Autodesk Inventor part; units mm, degrees
ref_plane "YZ Plane" through (0, 0, 0) normal (1, 0, 0) x (0, 1, 0)
ref_plane "XZ Plane" through (0, 0, 0) normal (0, 1, 0) x (-1, 0, 0)
ref_plane "XY Plane" through (0, 0, 0) normal (0, 0, 1) x (1, 0, 0)
sketch "Szkic1" plane through (0, 0, 0) normal (0, 1, 0) x (-1, 0, 0)
  line L0 (-125.2393, -14.1807) -> (-26.2247, 164.0455)
  arc A0 (-125.2393, -14.1807) -> (-99.0146, -58.75) centre (-99.0146, -28.75) ccw
  line L1 (99.0146, -58.75) -> (-99.0146, -58.75)
  line L2 (26.2247, 164.0455) -> (125.2393, -14.1807)
  arc A1 (26.2247, 164.0455) -> (-26.2247, 164.0455) centre (0, 149.4762) ccw
  line L3 (-23.6022, 162.5886) -> (-122.6168, -15.6376)
  arc A2 (-122.6168, -15.6376) -> (-99.0146, -55.75) centre (-99.0146, -28.75) ccw
  line L4 (-99.0146, -55.75) -> (99.0146, -55.75)
  arc A3 (113.6938, -51.4109) -> (125.9544, -30.5508) centre (99.0146, -28.75) ccw
  line L5 (122.6168, -15.6376) -> (23.6022, 162.5886)
  arc A4 (23.6022, 162.5886) -> (-23.6022, 162.5886) centre (0, 149.4762) ccw
  circle A5 centre (99.0146, -28.75) radius 5.1
  arc A6 (104.1146, -20.1483) -> (94.9151, -37.8711) centre (99.0146, -28.75) ccw
  line L6 (104.1146, -20.1483) -> (125.9544, -30.5508)
  line L7 (94.9151, -37.8711) -> (113.6938, -51.4109)
  arc A7 (99.0146, -58.75) -> (116.2857, -53.2797) centre (99.0146, -28.75) ccw
  arc A8 (128.8458, -31.9279) -> (125.2393, -14.1807) centre (99.0146, -28.75) ccw
  point P0 (0, 0)
  point P1 (0, 0)
  dimension "d0" = 3
  dimension "d1" = 10.2
  dimension "d2" = 20
extrude "Wyciągnięcie proste1" add sketch "Szkic1" along normal blind 5
sketch "Szkic2" plane through (0, 5, 0) normal (0, 1, 0) x (1, 0, 0)
  circle A0 centre (-99.0146, 28.75) radius 5.1
  circle A1 centre (-99.0146, 28.75) radius 5.1
  point P0 (0, 0)
extrude "Wyciągnięcie proste2" add sketch "Szkic2" against normal blind 5
sketch "Szkic3" plane through (0, 5, 0) normal (0, 1, 0) x (1, 0, 0)
  arc A0 (-104.1146, 20.1483) -> (-94.9151, 37.8711) centre (-99.0146, 28.75) ccw
  circle A1 centre (-99.0146, 28.75) radius 5.1
  circle A2 centre (-99.0146, 28.75) radius 10
  point P0 (0, 0)
  point P1 (-94.9151, 37.8711)
  dimension "d7" = 10.2
extrude "Wyciągnięcie proste3" add sketch "Szkic3" along normal blind 1
fillet "Zaokrąglenie1" radius 2 1 edges at (-107.8901, 5, -33.357)
sketch "Szkic4" plane through (0, 0, 0) normal (0, -1, 0) x (1, 0, 0)
  line L0 (-94.9151, -37.8711) -> (-113.6938, -51.4109)
  arc A0 (-94.9151, -37.8711) -> (-104.1146, -20.1483) centre (-99.0146, -28.75) ccw
  line L1 (-125.9544, -30.5508) -> (-104.1146, -20.1483)
  arc A1 (-125.9544, -30.5508) -> (-113.6938, -51.4109) centre (-99.0146, -28.75) ccw
  point P0 (0, 0)
extrude "Wyciągnięcie proste4" add sketch "Szkic4" along normal blind 15
properties part number "_Drukowanie 3D"
The listing builds one solid part. Answer for the finished solid, in the listing's coordinates (mm). A direction names the side the tool comes from. Coordinates: 2 decimals unless noted, no trailing zeros. Loops run counter-clockwise (first coordinate to the right, second up) from the corner with the lowest first, then second, coordinate; pieces in that order, holes last.
1) Find section C-C on y = -7. Write down the section's boundary in (x, z).
2) Find section A-A on z = -28.75. Write down the section's boundary in (x, y).
3) Find section B-B on x = -117.5. Write down the section's boundary in (y, z).
4) A tool of negligible diameter and unlimited length cuts with its end or side. For faces 4 (the face through (-104.173, -4.647, -44.546)), 5 (the face through (-99, 5, -29)), from which of +Z, -Z, +X, -X, +Y, -Y can it reach the whole face along a straight path? Write none if from no direction.
5) Determine the mould class of faces 1 (the face through (-115, 5, -37)), 2 (the face through (-114.882, -4.647, -25.277)), 3 (the face through (-108, -15, -35)) for opening direction Y: pulls with the +Y half, pulls with the -Y half, needs draft (parallel to the pull), parting line crosses it, or undercut.
6) Find the intervals of material crossed by L1, parallel to Y at x = -113.5, z = -29.5; L2, parallel to X at y = 5.7, z = -28.75; L3, parallel to X at y = 5.5, z = -28.75, in increasing order.
7) Find section D-D on z = -41. Write down the section's boundary in (x, y), then the cut area to 3 significant figures.
8) Flat-ended cylindrical pins translate along their axes: pin 1 Ø2 at (y, z) = (-8.5, -43.5) entering from +X; pin 2 Ø3 at (x, y) = (-93, 2.5) entering from +Z; pin 3 Ø3 at (x, z) = (-98.5, -29) entering from +Y. Find the tip coordinate at first contact, or state that the pin passes through.
Values:
1. outline: (-125.95, -30.55) arc R27 ccw to (-113.69, -51.41) - (-94.92, -37.87) arc R10 ccw (long way) to (-104.11, -20.15) - close
2. outline: (-122.17, -15) - (-89.01, -15) - (-89.01, 6) - (-93.91, 6) - (-93.91, 5) - (-104.11, 5) - (-104.11, 6) - (-109.01, 6) arc R2 cw to (-110.75, 5) - (-122.17, 5) - close
3. outline: (-15, -48.43) - (5, -48.43) - (5, -26.52) - (-15, -26.52) - close
4. face 4: -Z, +X, +Y, -Y
4. face 5: +Y
5. face 1: pulls with the +Y half
5. face 2: needs draft
5. face 3: pulls with the -Y half
6. L1: y = -15 to 5
6. L2: x = -109.23 to -104.11, -93.91 to -89.01
6. L3: x = -109.42 to -104.11, -93.91 to -89.01
7. outline: (-123.08, -15) - (-99.25, -15) - (-99.25, 5) - (-123.08, 5) - close
7. area: 476 mm2
8. pin 1: stops at x = -101.34
8. pin 2: stops at z = -19.83
8. pin 3: stops at y = 5
